Read the model definition and answer for the solid it produces. Units are mm, in the model's axes. A direction names the side the tool comes from. Coordinates: 2 decimals unless noted, no trailing zeros. Order: outer loops, then holes, each group sorted by start corner. A loop starts at its lowest first (then second) coordinate and runs counter-clockwise, first axis right, second up. Notation, with made-up numbers: (41.5, 5.25) -> (93.5, 5.25) arc R26 cw to (93.5, 42.25) -> close; hole circle Ø2 at (-15.75, -8.75). An arc over 180 degrees is marked (long way). Answer as a JSON object with one key per item and string values. Group by question number.
1) Section B-B on z = -17.5 is taken. Determine the outline of the cut face in (x, y).
2) Given pin 1 (1.4 mm diameter, centred on x = -7.04, z = -12.2, fed in from -Y); pin 2 (2 mm diameter, centred on x = 0.5, z = 0.5, fed in from +Y); pin 3 (1.3 mm diameter, centred on x = 0, z = -12.2, fed in from +Y), each flat-ended and moving along its own axis, determine where each tip first touches the part or whether it passes through.
3) Determine the mould class of faces 1 (the conical face through (-6.902, 31.403, -12.218)), 2 (the flat face through (0, 0, 0)), 3 (the flat face through (0, 16, -23.8)) for opening direction Z: released by +Z, released by -Z, zero draft, split by the parting line, or undercut.
4) Section C-C on y = 35.5 is taken. Determine the outline of the cut face in (x, z).
5) Consider L1, parallel to X at y = 33.35, z = -12.2; L2, parallel to X at y = 34, z = -12; L3, parallel to Y at x = -4, z = 10. Determine where each line is inside the solid, lowest interval first.
6) Section D-D on z = 6 is taken. Determine the outline of the cut face in (x, y), and give its area (3 significant figures).
7) A tool of negligible diameter and unlimited length cuts with its end or side. For faces 4 (the flat face through (0, 16, 23.8)), 5 (the cylindrical face through (0, 34, -13)), from which of +Z, -Z, +X, -X, +Y, -Y can it reach the whole face along a straight path? Write none if from no direction.
8) Section A-A on x = -5.5 is taken. Determine the outline of the cut face in (y, z), and give its area (3 significant figures).
from build123d import *

# Parameters (mm, degrees)
SKETCH1_W                 = 26.2
SKETCH1_H                 = 47.6
BOSS_EXTRUDE1_DEPTH       = 32
SKETCH2_R                 = 11.6
BOSS_EXTRUDE2_DEPTH       = 5
M2X0_4_TAPPED_HOLE1_D     = 1.6
M2X0_4_TAPPED_HOLE1_DEPTH = 5.2
M2X0_4_TAPPED_HOLE1_TIP   = 0.480688495


with BuildPart() as part:
    # Sketch1 → Boss-Extrude1 (new body)
    with BuildSketch(Plane(origin=(0, 0, 0), x_dir=(1, 0, 0), z_dir=(0, 1, 0))):
        Rectangle(SKETCH1_W, SKETCH1_H)
    extrude(amount=BOSS_EXTRUDE1_DEPTH)

    # Sketch2 → Boss-Extrude2 (add)
    with BuildSketch(Plane(origin=(0, 32, 0), x_dir=(-1, 0, 0), z_dir=(0, 1, 0))):
        with Locations(Location((0, -12.2, 0), (0, 0, 270))):
            Circle(SKETCH2_R)
    extrude(amount=BOSS_EXTRUDE2_DEPTH)

    # M2x0.4 Tapped Hole1
    with Locations(Plane(origin=(0, 37, -12.2), x_dir=(0, 0, 1), z_dir=(0, 1, 0))):
        with Locations((0, 0), (0, -7.039859919), (0, 7.136767925)):
            Hole(M2X0_4_TAPPED_HOLE1_D / 2, depth=M2X0_4_TAPPED_HOLE1_DEPTH)
            with Locations((0, 0, -(M2X0_4_TAPPED_HOLE1_DEPTH + M2X0_4_TAPPED_HOLE1_TIP / 2))):  # 118° drill point
                Cone(0, M2X0_4_TAPPED_HOLE1_D / 2, M2X0_4_TAPPED_HOLE1_TIP, mode=Mode.SUBTRACT)


solid = part.part
Worked answers:
{
 "1": {"outline": "(-13.1, 0) -> (13.1, 0) -> (13.1, 32) -> (10.32, 32) -> (10.32, 37) -> (-10.32, 37) -> (-10.32, 32) -> (-13.1, 32) -> close"},
 "2": {"pin 1": "stops at y = 0", "pin 2": "stops at y = 32", "pin 3": "stops at y = 31.71"},
 "3": {"face 1": "undercut", "face 2": "zero draft", "face 3": "released by -Z"},
 "4": {"outline": "circle Ø23.2 at (0, -12.2); hole circle Ø1.6 at (-7.04, -12.2); hole circle Ø1.6 at (0, -12.2); hole circle Ø1.6 at (7.14, -12.2)"},
 "5": {"L1": "x = -11.6 to -7.84, -6.24 to -0.8, 0.8 to 6.34, 7.94 to 11.6", "L2": "x = -11.6 to -7.81, -6.27 to -0.77, 0.77 to 6.36, 7.91 to 11.6", "L3": "y = 0 to 32"},
 "6": {"outline": "(-13.1, 0) -> (13.1, 0) -> (13.1, 32) -> (-13.1, 32) -> close", "area": "838 mm²"},
 "7": {"face 4": "+Z, +X, -X, +Y, -Y", "face 5": "+Y"},
 "8": {"outline": "(0, -23.8) -> (32, -23.8) -> (32, -22.41) -> (37, -22.41) -> (37, -1.99) -> (32, -1.99) -> (32, 23.8) -> (0, 23.8) -> close", "area": "1,630 mm²"}
}
